Autodesk Fusion 360 part; units mm, degrees
sketch "Sketch1" plane through (0, 0, 0) normal (0, 0, 1) x (1, 0, 0)
  circle A0 centre (-2.9141, 22.4848) radius 1.25
  line L0 (-9, 12) -> (-9, 31)
  arc A1 (9, -12) -> (9, 12) centre (0, 0) ccw
  arc A2 (-10.5, -25) -> (10.5, -25) centre (0, -25) ccw
  line L1 (0, 0) -> (0, 12) construction
  circle A3 centre (0, 0) radius 3
  arc A4 (9, 31) -> (-9, 31) centre (0, 31) ccw
  arc A5 (10.5, -12.7279) -> (10.5, 12.7279) centre (0, 0) ccw
  circle A6 centre (0, 31) radius 1.25
  line L2 (-10.5, -25) -> (-10.5, -12.7279)
  arc A7 (-9, 12) -> (-9, -12) centre (0, 0) ccw
  line L3 (9, -25) -> (9, -12)
  circle A8 centre (0, 0) radius 12 construction
  circle A9 centre (-2.9141, 22.4848) radius 2.5 construction
  line L4 (10.5, -25) -> (10.5, -12.7279)
  circle A10 centre (0, 14.5) radius 2.5 construction
  arc A11 (-9, -25) -> (9, -25) centre (0, -25) ccw
  line L5 (-9, -25) -> (-9, -12)
  line L6 (0, -25) -> (0, 0) construction
  arc A12 (10.5, 31) -> (-10.5, 31) centre (0, 31) ccw
  circle A13 centre (0, 14.5) radius 6 construction
  line L7 (10.5, 12.7279) -> (10.5, 31)
  line L8 (-10.5, 12.7279) -> (-10.5, 31)
  circle A14 centre (0, 14.5) radius 1.25
  line L9 (0, 14.5) -> (0, 12) construction
  arc A15 (-10.5, 12.7279) -> (-10.5, -12.7279) centre (0, 0) ccw
  line L10 (-9, 21.5) -> (-10.5, 21.5) construction
  line L11 (-6, 23) -> (-9, 23) construction
  circle A16 centre (0, 31) radius 4.5 construction
  line L12 (9, 12) -> (9, 31)
  circle A17 centre (-2.9141, 22.4848) radius 4.5 construction
  line L13 (9, 21.5) -> (10.5, 21.5) construction
  line L14 (9, 27.5) -> (10.5, 27.5)
  line L15 (9, 23) -> (10.5, 23) construction
  line L16 (9, 23) -> (6, 23) construction
  circle A18 centre (6, 23) radius 2
  arc A19 (9.75, 31) -> (-9.75, 31) centre (0, 31) ccw
  line L17 (-9.75, 12.3693) -> (-9.75, 31)
  arc A20 (-9.75, 12.3693) -> (-9.75, -12.3693) centre (0, 0) ccw
  line L18 (-9.75, -25) -> (-9.75, -12.3693)
  arc A21 (-9.75, -25) -> (9.75, -25) centre (0, -25) ccw
  line L19 (9.75, -25) -> (9.75, -18.5)
  line L20 (9.75, 27.5) -> (9.75, 31)
  line L21 (9, -18.5) -> (10.5, -18.5)
  circle A22 centre (6, 23) radius 1.375
  circle A23 centre (0, 0) radius 2
  circle A24 centre (0, -25) radius 2
  circle A25 centre (0, -25) radius 1.375
  circle A26 centre (0, 14.5) radius 1.75
  circle A27 centre (-2.9141, 22.4848) radius 1.75
  dimension "d1" = 1.5
  dimension "d3" = 56
  dimension "d4" = 30
  dimension "d5" = 18
  dimension "d6" = 18
  dimension "d7" = 6
  dimension "d8" = 24
  dimension "d9" = 25
  dimension "d10" = 12
  dimension "d11" = 5
  dimension "d12" = 9
  dimension "d13" = 5
  dimension "d14" = 9
  dimension "d15" = 15
  dimension "d16" = 2.5
  dimension "d17" = 2.5
  dimension "d18" = 2.5
  dimension "d19" = 3
  dimension "d20" = 8
  dimension "d28" = 6
  dimension "d29" = 8
  dimension "d30" = 3
  dimension "d31" = 4
  dimension "d33" = 3.5
  dimension "d34" = 15.75
  dimension "d35" = 2.75
  dimension "d36" = 4
  dimension "d37" = 2.75
  dimension "d38" = 4
  dimension "d47" = 3.5
  dimension "d48" = 3.5
extrude "Extrude1" add sketch "Sketch1" along normal blind 1 contours L0 A1 A4 A7 L3 A11 L5 L12 | A1 A5 L3 L4 L7 L12 L14 L21 | A26 | A27
extrude "Extrude4" add sketch "Sketch1" along normal blind 2 contours A1 A5 L3 L4 L7 L12 L14 L21
extrude "Extrude5" add sketch "Sketch1" along normal blind 1.95 contours A0 | A14 | A26 | A27
extrude "Extrude6" add sketch "Sketch1" along normal blind 2.95 contours A18 | A22
extrude "Extrude7" add sketch "Sketch1" along normal blind 3.95 contours A22
extrude "Extrude8" add sketch "Sketch1" along normal blind 1 contours A3 | A23
extrude "Extrude9" add sketch "Sketch1" along normal blind 1.95 contours A24 | A25
extrude "Extrude10" cut sketch "Sketch1" along normal blind 1.5 from surface at 1 contours A25
extrude "Extrude2" add sketch "Sketch1" along normal blind 3 contours A2 L2 L4 A12 L7 L8 A15 L14 A19 L17 A20 L18 A21 L19 L20 L21
extrude "Extrude3" add sketch "Sketch1" along normal blind 4 contours L0 A4 A7 L3 A11 L5 L12 L14 A19 L17 A20 L18 A21 L19 L20 L21
fillet "Fillet1" radius 0.25 9 edges at (9, 27.5, 3) (-10.5, -18.864, 0) (0, -35.5, 0) (10.5, -18.864, 0) (16.5, 0, 0) (10.5, 21.864, 0) (0, 41.5, 0) (-10.5, 21.8639, 0) (-16.5, 0, 0)
equation "d6 = d5"
Read the model definition and answer for the solid it produces. Units are mm, in the model's axes. A direction names the side the tool comes from. Round coordinates to 2 decimals unless told otherwise and drop trailing zeros. Order: outer loops, then holes, each group sorted by start corner. A loop starts at its lowest first (then second) coordinate and runs counter-clockwise, first axis right, second up. Notation, with made-up numbers: (68.5, 81.25) - (88.5, 81.25) arc R22 ccw to (88.5, 100.25) - close; hole circle Ø7 at (62.5, -1.75). An arc over 180 degrees is marked (long way). Use one line per item in the form item = value. Start each with the question number.
(1) For faces 1 (the face through (14.4, 4.73, 2)), 2 (the face through (0.214, -34.748, 3.493)), 3 (the face through (0, 40, 2)), 4 (the face through (-10.5, 22, 2)), determine the directions among +Z, -Z, +X, -X, +Y, -Y from which every point of the face is accessible in a straight line to the end or side of a thin tool.
(2) Determine the mould class of faces 5 (the face through (15, 0.2, 1.5)), 6 (the face through (16.5, 0.2, 1.1)), 7 (the face through (-16.5, -0.2, 1.6)) for opening direction X: +X half, -X half, draft (parallel to the pull), parting line (faces both ways), or undercut.
(3) Find the intervals of material crossed by line 1 along Y through (x, z) = (0, 1.75) (3 decimals); line 2 along Y through (x, z) = (0, 0.85); line 3 along X through (y, z) = (16.5, 1.7), in increasing order. Write a range as from..to.
(4) Flat-ended cylindrical pins translate along their axes: pin 1 Ø0.9 at (y, z) = (-16.5, 2.5) entering from -X; pin 2 Ø2 at (x, y) = (14.5, -4) entering from +Z; pin 3 Ø5 at (x, y) = (-2.5, 7) entering from -Z; pin 4 Ø8 at (x, y) = (-0.5, 4) entering from +Z. Find the tip coordinate at first contact, or state that the pin passes through.
(5) The part is cut by section A-A (y = 14.5). Give the vertices of the cut face in (x, z), then the cut area to 3 significant figures.
Checked values:
q1.face_1 = +Z, +X
q1.face_2 = +Z, -Y
q1.face_3 = +Z
q1.face_4 = +Z, -Z, -X, +Y
q2.face_5 = undercut
q2.face_6 = +X half
q2.face_7 = -X half
q3.line_1 = -35.5..-34, -27..-26.375, -23.625..-23, 12.75..16.25, 40..41.5
q3.line_2 = -35.5..29.75, 32.25..41.5
q3.line_3 = -10.5..-9, 9..10.5
q4.pin_1 = -10.5
q4.pin_2 = 2
q4.pin_3 = 0
q4.pin_4 = 1
q5.outline = (-10.5, 0.25) arc R0.25 ccw to (-10.25, 0) - (10.25, 0) arc R0.25 ccw to (10.5, 0.25) - (10.5, 2) - (9, 2) - (9, 1) - (1.75, 1) - (1.75, 1.95) - (-1.75, 1.95) - (-1.75, 1) - (-9, 1) - (-9, 4) - (-9.75, 4) - (-9.75, 3) - (-10.5, 3) - close
q5.area = 29.5 mm^2
